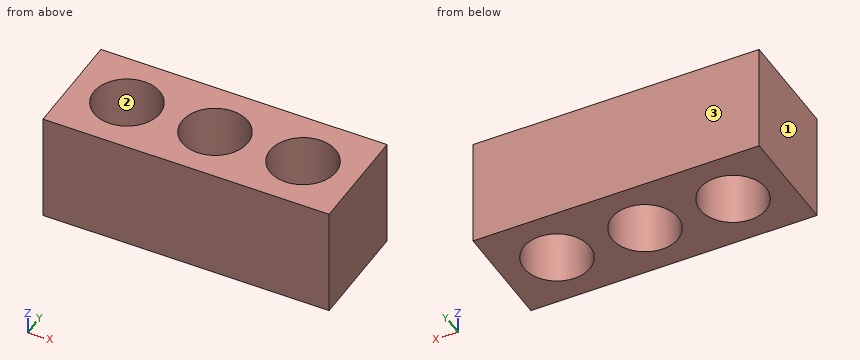
from build123d import *

# Parameters (mm, degrees)
F0_W     = 41.275
F0_H     = 15.875
F0_R     = 4.7625
F1_DEPTH = 15.875
F2_ANGLE = 90


with BuildPart() as f1:
    # F0 (on Front) → F1 (new body)
    with BuildSketch(Plane.XZ):
        Rectangle(F0_W, F0_H)
        with Locations((-12.7, 0)):
            Circle(F0_R, mode=Mode.SUBTRACT)
        Circle(F0_R, mode=Mode.SUBTRACT)
        with Locations((12.7, 0)):
            Circle(F0_R, mode=Mode.SUBTRACT)
    extrude(amount=-F1_DEPTH)


with BuildPart() as f1_1:
    # F2: moved
    add(f1.part.rotate(Axis((6.35, 0, 0), (1, 0, 0)), F2_ANGLE))


solid = f1_1.part
Geometry: final body of the model. Coordinates: model frame, mm. Face numbers are marked on the shaded views. Give positions to 0.01 mm unless a question says otherwise; leave off trailing zeros. Write each loop counter-clockwise with the first axis right and the second up, starting at its lowest first coordinate (ties: lowest second). Pieces come first, ordered by that corner, then holes.
(1) Ray query, line 1 (X direction, y = 0, z = 4); line 2 (Y direction, x = 12.7, z = 10.5); line 3 (X direction, y = 0.5, z = 8). Return the intervals inside material, ascending.
(2) Cut plane C-C, the plane y = 0. Return loops of the section in (x, z) (1 decimal), then the cut area to 3 significant figures.
(3) First-contact query: P1, Ø5.5, axis at x = 0, y = 0, coming from the +Z side. Flat tip, straight axial feed; report the tip coordinate or a pass-through.
(4) Cut plane B-B, the plane z = 7.5. Return loops of the section in (x, y) (1 decimal).
(5) Cut plane A-A, the plane x = 0. Return loops of the section in (y, z) (1 decimal), then the cut area to 3 significant figures.
(6) Mould query, pull axis X, two halves, no side actions, for the marked faces 1, 2 and 3. Classes: released by +X, released by -X, zero draft, split by the parting line, or undercut.
Values follow:
1. line 1: x = -20.64 to -17.46, -7.94 to -4.76, 4.76 to 7.94, 17.46 to 20.64
1. line 2: y = -7.94 to -4.76, 4.76 to 7.94
1. line 3: x = -20.64 to -17.44, -7.96 to -4.74, 4.74 to 7.96, 17.44 to 20.64
2. outline: (-20.6, 0) - (-17.5, 0) - (-17.5, 15.9) - (-20.6, 15.9) - close; (-7.9, 0) - (-4.8, 0) - (-4.8, 15.9) - (-7.9, 15.9) - close; (4.8, 0) - (7.9, 0) - (7.9, 15.9) - (4.8, 15.9) - close; (17.5, 0) - (20.6, 0) - (20.6, 15.9) - (17.5, 15.9) - close
2. area: 202 mm2
3. P1: passes through
4. outline: (-20.6, -7.9) - (20.6, -7.9) - (20.6, 7.9) - (-20.6, 7.9) - close; hole circle Ø9.5 at (-12.7, 0); hole circle Ø9.5 at (0, 0); hole circle Ø9.5 at (12.7, 0)
5. outline: (-7.9, 0) - (-4.8, 0) - (-4.8, 15.9) - (-7.9, 15.9) - close; (4.8, 0) - (7.9, 0) - (7.9, 15.9) - (4.8, 15.9) - close
5. area: 101 mm2
6. face 1: released by -X
6. face 2: undercut
6. face 3: zero draft
